Read the model definition and answer for the solid it produces. Units are mm, in the model's axes. Coordinates: 2 decimals unless noted, no trailing zeros. Write each loop counter-clockwise with the first axis right and the second up, starting at its lowest first coordinate (ties: lowest second). Pieces come first, ordered by that corner, then holes. Notation, with made-up numbers: (-16.5, 71.5) -> (10.5, 71.5) arc R30 ccw to (10.5, 93.5) -> close; hole circle Ø10 at (67, -9). An arc over 180 degrees is marked (long way). One line per item, written item: value. Start each with the question number.
1. Consider line 1 along Y through (x, z) = (24, 1.3); line 2 along Z through (x, y) = (59, 1); line 3 along Z through (x, y) = (48, 2.75). Determine where each line is inside the solid, lowest interval first.
2. Given P1, Ø7.5, axis at x = 48, y = -4, coming from the -Z side; P2, Ø3, axis at x = 8, y = -4, coming from the -Z side, each flat-ended and moving along its own axis, determine where each tip first touches the part or whether it passes through.
3. Find section A-A, the plane x = 16. Write down the section's boundary in (y, z), and give its area (3 significant figures).
```python
from build123d import *

# Parameters (mm, degrees)
F1_DEPTH  = 8
F3_W      = 8
F3_H      = 8
F3_R      = 2.4
F4_DEPTH  = 1.7
F5_R      = 2.4
F6_DEPTH  = 1.7
F15_W     = 30.2577763796
F15_H     = 33.55890885
F16_DEPTH = 48.006


with BuildPart() as f1:
    # F0 (on Front) → F1 (new body)
    with BuildSketch(Plane.XZ):
        Polygon((-2.4, 9.6), (-4, 9.6), (-4, 0), (4, 0), (4, 9.6), (2.4, 9.6), (2.4, 11.3), (-2.4, 11.3), align=None)
    extrude(amount=F1_DEPTH)

    # F3 (on plane+point) → F4 (cut, through all)
    with BuildSketch(Plane.XY.offset(11.3)):
        with Locations((0, -4)):
            Rectangle(F3_W, F3_H)
        with Locations((0, -4)):
            Circle(F3_R, mode=Mode.SUBTRACT)
    extrude(amount=-F4_DEPTH, mode=Mode.SUBTRACT)

    # F5 (on Top) → F6 (cut)
    with BuildSketch(Plane.XY):
        with Locations((0, -4)):
            Circle(F5_R)
    extrude(amount=F6_DEPTH, mode=Mode.SUBTRACT)

    # F8: F1 across plane


with BuildPart() as f1_1:
    add(f1.part)
    add(f1.part.mirror(Plane.YZ.offset(4)))

    # F9: F1 across plane


with BuildPart() as f1_2:
    add(f1_1.part)
    add(f1_1.part.mirror(Plane.XZ))

    # F11: F1 across plane


with BuildPart() as f1_3:
    add(f1_2.part)
    add(f1_2.part.mirror(Plane.YZ.offset(12)))

    # F12: F1 across face


with BuildPart() as f1_4:
    add(f1_3.part)
    add(f1_3.part.mirror(Plane(origin=(28, 0, 4.8), x_dir=(0, 1, 0), z_dir=(1, 0, 0))))

    # F13: F1 across face


with BuildPart() as f1_5:
    add(f1_4.part)
    add(f1_4.part.mirror(Plane(origin=(60, 0, 4.8), x_dir=(0, 1, 0), z_dir=(1, 0, 0))))

    # F15 (on offset) → F16 (cut)
    with BuildSketch(Plane.YZ.offset(124)):
        with Locations((0, 4.603235051)):
            Rectangle(F15_W, F15_H)
    extrude(amount=-F16_DEPTH, mode=Mode.SUBTRACT)


solid = f1_5.part
```
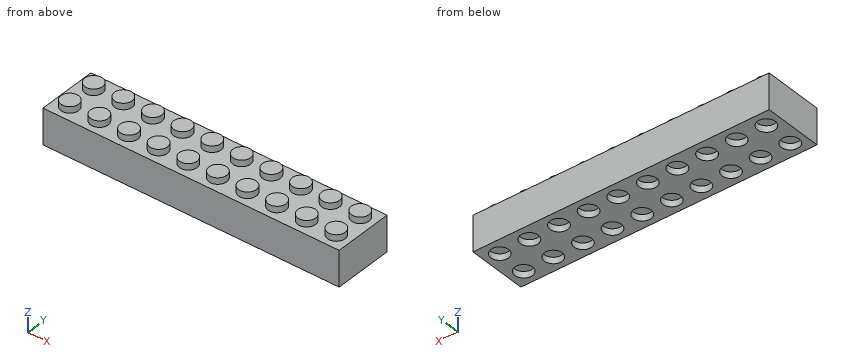
Answer block:
1. line 1: y = -8 to -6.4, -1.6 to 1.6, 6.4 to 8
1. line 2: z = 0 to 9.6
1. line 3: z = 1.7 to 11.3
2. P1: stops at z = 0
2. P2: stops at z = 1.7
3. outline: (-8, 0) -> (-6.4, 0) -> (-6.4, 1.7) -> (-1.6, 1.7) -> (-1.6, 0) -> (1.6, 0) -> (1.6, 1.7) -> (6.4, 1.7) -> (6.4, 0) -> (8, 0) -> (8, 9.6) -> (6.4, 9.6) -> (6.4, 11.3) -> (1.6, 11.3) -> (1.6, 9.6) -> (-1.6, 9.6) -> (-1.6, 11.3) -> (-6.4, 11.3) -> (-6.4, 9.6) -> (-8, 9.6) -> close
3. area: 154 mm2
